Model file for the job. Use its own axes, mm. A direction names the side the tool comes from. Give positions to 0.01 mm unless a question says otherwise; leave off trailing zeros. Answer as a JSON object with one key per item and string values. Group by question number.
```python
from build123d import *

# Parameters (mm, degrees)
F0_W = 2
F0_H = 0.675


with BuildPart() as f1:
    # F0 (on Front) → F1 (revolve)
    with BuildSketch(Plane.XZ):
        with Locations((0, 0.6625)):
            Rectangle(F0_W, F0_H)
        with BuildLine():
            add(Edge.make_bspline(
                [(25.2, 4), (20.2, 4), (12.59111, 4.105829), (1, 1)],
                knots=[0, 0, 0, 0, 24.385241, 24.385241, 24.385241, 24.385241], degree=3))
            Line((1, 1), (1, 0.325))
            add(Edge.make_bspline(
                [(25.2, 3.275), (20.2, 3.424434), (12.59111, 3.302944), (1, 0.325)],
                knots=[0, 0, 0, 0, 24.379141, 24.379141, 24.379141, 24.379141], degree=3))
            Line((25.2, 3.275), (25.2, 4))
        make_face()
        Polygon((30.2, 4), (25.2, 4), (25.2, 3.275), (27.7, 3.275), (30.2, 3.275), align=None)
    revolve(axis=Axis((13.85, 0, 0), (1, 0, 0)))

    # F2 (on Top) → F3 (revolve)
    with BuildSketch(Plane.XY):
        Polygon((20.365128, -3.429), (15.875, -3.175), (12.314808, -6.735192), (14.542194, -8.962578), (10.228843, -13.27593), (10.741495, -13.788582), (16.242975, -8.287103), (15.875, -7.919128), align=None)
    revolve(axis=Axis((12.314808, -6.735192, 0), (-0.707107, -0.707107, 0)))

    # F4 (on Front) → F5 (revolve, cut)
    with BuildSketch(Plane.XZ):
        with BuildLine():
            Line((27.7, 0), (27.7, 3.275))
            Line((27.7, 3.275), (25.2, 3.275))
            add(Edge.make_bspline(
                [(25.2, 3.275), (20.2, 3.424434), (12.59111, 3.302944), (1, 0.325)],
                knots=[0, 0, 0, 0, 24.379141, 24.379141, 24.379141, 24.379141], degree=3))
            Line((1, 0.325), (1, 0))
            Line((1, 0), (27.7, 0))
        make_face()
    revolve(axis=Axis((13.85, 0, 0), (1, 0, 0)), mode=Mode.SUBTRACT)


solid = f1.part
```
Q1. Drop flat-ended pins along their axis: P1, Ø1, axis at x = 3.5, z = -1.5, coming from the -Y side; P2, Ø4, axis at x = 10.5, z = 0, coming from the +Y side. Give the stop position or say it passes through.
Q2. Wall check: L1, parallel to Z at x = -0.5, y = 0 (3 decimals); L2, parallel to Y at x = 27.05, z = 0 (3 decimals). Give the ranges that are in metal, low to high.
Q3. Two-plate mould, pull along X, no slides. Class faces 4 (the flat face through (-1, 0.21, -0.43)), 5 (the flat face through (30.2, 3, 2)), 6 (the flat face through (12.35, -6.77, 0.04)): +X half, -X half, draft (parallel to the pull), parting line (faces both ways), or undercut.
Q4. Slice it at A-A, the plane z = 0. Count the separate pieces of the cut face and the enclosed holes in it, then the cut area to 3 significant figures.
Q5. 3-axis set-ups, long thin cutter, end or side, ignore diameter. For faces 1 (the cylindrical face through (12.055, -9.524, -3.438)), 2 (the cylindrical face through (0, 1, 0)), 3 (the cylindrical face through (27.665, 3.905, -0.867)): which of +Z, -Z, +X, -X, +Y, -Y reach the whole face in a straight line?
Solved:
{
 "1": {"P1": "stops at y = -1.32", "P2": "stops at y = 3.32"},
 "2": {"L1": "z = -1 to -0.325, 0.325 to 1", "L2": "y = -4 to -3.275, 3.275 to 4"},
 "3": {"face 4": "-X half", "face 5": "+X half", "face 6": "undercut"},
 "4": {"separate pieces": "2", "enclosed holes": "1", "area": "83.8 mm²"},
 "5": {"face 1": "none", "face 2": "-X", "face 3": "+X"}
}
